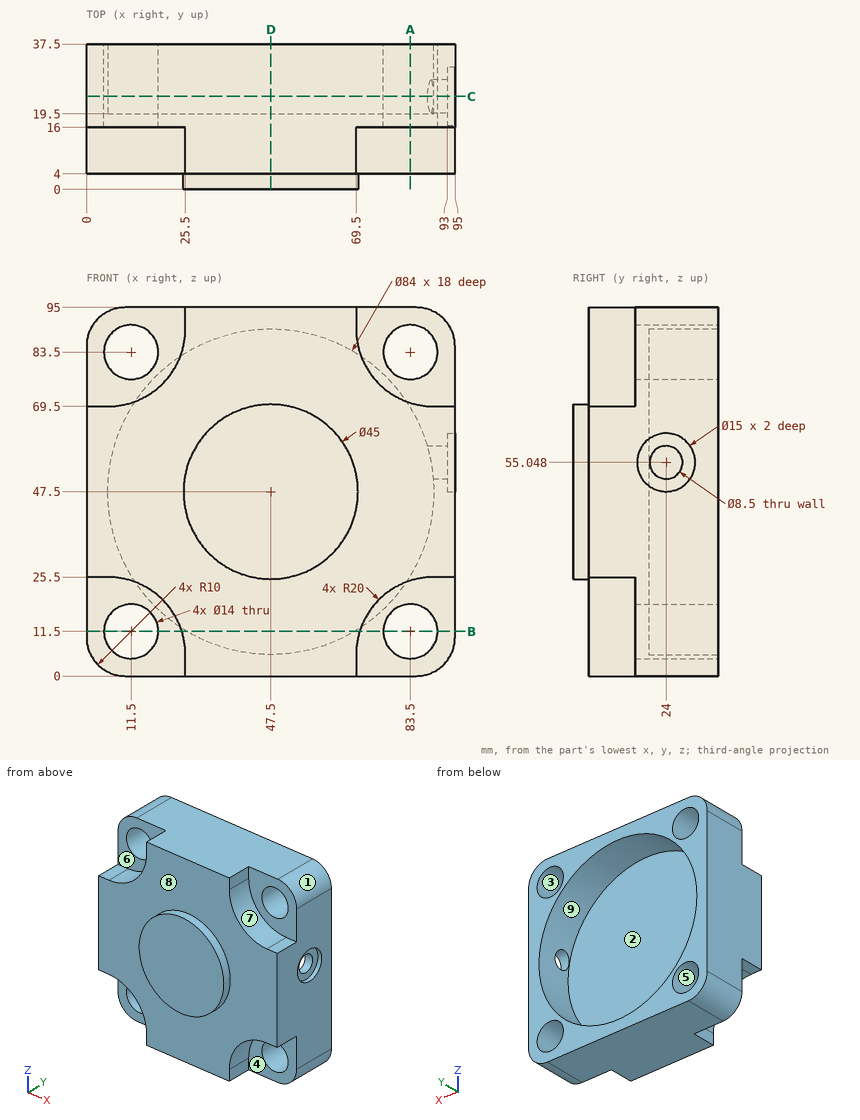
Source: three-view drawing plus pictorial views. Frame: mm from the lowest corner of the part. A direction names the side the tool comes from. Give positions to 0.01 mm unless a question says otherwise; leave off trailing zeros. Order: outer loops, then holes, each group sorted by start corner. A loop starts at its lowest first (then second) coordinate and runs counter-clockwise, first axis right, second up. Notation, with made-up numbers: (5, 22) - (23, 22) arc R27 cw to (23, 57) - close; hole circle Ø4 at (-5, 20.25). An arc over 180 degrees is marked (long way). Answer as a JSON object with one key per item and string values. Group by question number.
Q1. Line query: probe 1 along Z at (x, y) = (47.5, 27); probe 2 along Y at (x, z) = (9.5, 25). Output: solid intervals per line, ascending.
Q2. Mould query, pull axis Z, two halves, no side actions, for the marked faces 1, 2, 3 and 4. Classes: pulls with the +Z half, pulls with the -Z half, needs draft (parallel to the pull), parting line crosses it, or undercut.
Q3. First-contact query: pin 1 Ø1.5 at (x, z) = (44.5, 56) entering from +Y; pin 2 Ø10 at (y, z) = (7, 78) entering from -X; pin 3 Ø4.5 at (x, y) = (92.5, 12.5) entering from -Z; pin 4 Ø1.5 at (x, y) = (72, 32) entering from -Z. Flat tips, straight axial feed; report the tip coordinate or a pass-through.
Q4. Cut plane A-A, the plane x = 83.5. Output: boundary loops of the cut face in (y, z), then the cut area to 3 significant figures.
Q5. Set-up query: the marked faces 5, 6, 7, 8 and 9. Return all of +Z, -Z, +X, -X, +Y, -Y with unobstructed straight access to the full face (end or side cutting, diameter ignored); none if empty.
Q6. Cut plane C-C, the plane y = 24. Output: boundary loops of the cut face in (x, z).
Q7. Cut plane D-D, the plane x = 47.5. Output: boundary loops of the cut face in (y, z), then the cut area to 3 significant figures.
Q8. Cut plane B-B, the plane z = 11.5. Output: boundary loops of the cut face in (x, y).
Results:
{
 "1": {"probe 1": "0 to 5.5, 89.5 to 95", "probe 2": "16 to 37.5"},
 "2": {"face 1": "pulls with the +Z half", "face 2": "undercut", "face 3": "undercut", "face 4": "needs draft"},
 "3": {"pin 1": "y = 19.5", "pin 2": "x = 16.8", "pin 3": "z = 25.5", "pin 4": "z = 0"},
 "4": {"outline": "(4, 24.58) - (16, 24.58) - (16, 18.5) - (37.5, 18.5) - (37.5, 25.87) - (19.5, 25.87) - (19.5, 69.13) - (37.5, 69.13) - (37.5, 76.5) - (16, 76.5) - (16, 70.42) - (4, 70.42) - close; (16, 0) - (37.5, 0) - (37.5, 4.5) - (16, 4.5) - close; (16, 90.5) - (37.5, 90.5) - (37.5, 95) - (16, 95) - close", "area": "1,210 mm^2"},
 "5": {"face 5": "+Y, -Y", "face 6": "+Z, -X, -Y", "face 7": "+Z, +X, -Y", "face 8": "-Y", "face 9": "+Y"},
 "6": {"outline": "(0, 10) arc R10 ccw to (10, 0) - (85, 0) arc R10 ccw to (95, 10) - (95, 47.55) - (93, 47.55) - (93, 50.8) - (89.37, 50.8) arc R42 cw (long way) to (87.81, 59.3) - (93, 59.3) - (93, 62.55) - (95, 62.55) - (95, 85) arc R10 ccw to (85, 95) - (10, 95) arc R10 ccw to (0, 85) - close; hole circle Ø14 at (11.5, 11.5); hole circle Ø14 at (11.5, 83.5); hole circle Ø14 at (83.5, 11.5); hole circle Ø14 at (83.5, 83.5)"},
 "7": {"outline": "(0, 25) - (4, 25) - (4, 0) - (37.5, 0) - (37.5, 5.5) - (19.5, 5.5) - (19.5, 89.5) - (37.5, 89.5) - (37.5, 95) - (4, 95) - (4, 70) - (0, 70) - close", "area": "1,850 mm^2"},
 "8": {"outline": "(0, 16) - (4.5, 16) - (4.5, 37.5) - (0, 37.5) - close; (18.5, 16) - (24.58, 16) - (24.58, 4) - (70.42, 4) - (70.42, 16) - (76.5, 16) - (76.5, 37.5) - (69.13, 37.5) - (69.13, 19.5) - (25.87, 19.5) - (25.87, 37.5) - (18.5, 37.5) - close; (90.5, 16) - (95, 16) - (95, 37.5) - (90.5, 37.5) - close"}
}
